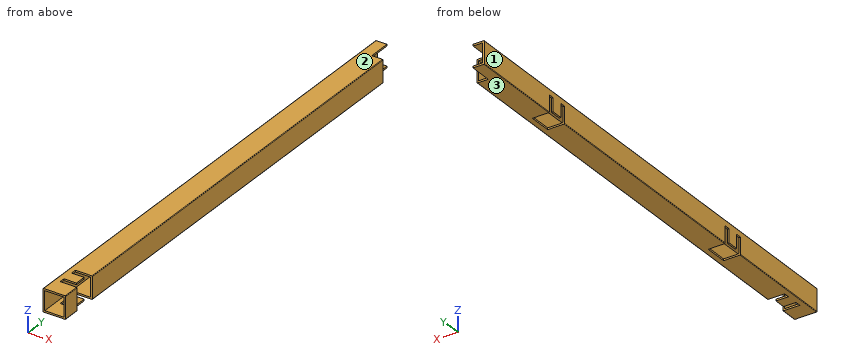
```python
from build123d import *

# Parameters (mm, degrees)
SKETCH1_W                   = 17
SKETCH1_H                   = 17
BOSS_EXTRUDE1_DEPTH         = 1220
SKETCH2_W                   = 20
SKETCH2_H                   = 20
CUT_EXTRUDE1_DEPTH          = 10
CUT_EXTRUDE2_DEPTH          = 15
SKETCH4_W                   = 3
SKETCH4_H                   = 10
CUT_EXTRUDE3_DEPTH          = 10
SKETCH_PATTERN1_START       = -20
SKETCH_PATTERN1_DEPTH       = 15
SKETCH_PATTERN1_2_OUTLINE_W = 1.5
SKETCH_PATTERN1_2_OUTLINE_H = 10
SKETCH_PATTERN1_2_DEPTH     = 3
SKETCH6_W                   = 20
SKETCH6_H                   = 20
CUT_EXTRUDE4_DEPTH          = 4
CUT_EXTRUDE5_DEPTH          = 1221.327824808
CUT_EXTRUDE5_DEPTH_BACK     = 1221.327824808
SKETCH7_W                   = 11
SKETCH7_H                   = 5
SKETCH8_W                   = 20.081282068
SKETCH8_H                   = 792.599518512
CUT_EXTRUDE6_DEPTH          = 20


# Read off the part's stored shape, not the designer's step: Sketch-Pattern1
with BuildPart() as part:
    # Sketch1 → Boss-Extrude1 (new body)
    with BuildSketch(Plane(origin=(0, 0, 0), x_dir=(1, 0, 0), z_dir=(0, 1, 0))):
        with BuildLine():
            Line((0.5, 0), (19.5, 0))
            ThreePointArc((19.5, 0), (19.853553391, 0.146446609), (20, 0.5))
            Line((20, 0.5), (20, 19.5))
            ThreePointArc((20, 19.5), (19.853553391, 19.853553391), (19.5, 20))
            Line((19.5, 20), (0.5, 20))
            ThreePointArc((0.5, 20), (0.146446609, 19.853553391), (0, 19.5))
            Line((0, 19.5), (0, 0.5))
            ThreePointArc((0, 0.5), (0.146446609, 0.146446609), (0.5, 0))
        make_face()
        with Locations((10, 10)):
            Rectangle(SKETCH1_W, SKETCH1_H, mode=Mode.SUBTRACT)
    extrude(amount=BOSS_EXTRUDE1_DEPTH)

    # Sketch2 → Cut-Extrude1 (cut)
    with BuildSketch(Plane(origin=(20, 0, 0), x_dir=(0, 0, -1), z_dir=(1, 0, 0))):
        with Locations((10, 1210)):
            Rectangle(SKETCH2_W, SKETCH2_H)
        with Locations((10, 10)):
            Rectangle(SKETCH2_W, SKETCH2_H)
    extrude(amount=-CUT_EXTRUDE1_DEPTH, mode=Mode.SUBTRACT)

    # Sketch3 → Cut-Extrude2 (cut)
    with BuildSketch(Plane(origin=(0, 0, -20), x_dir=(-1, 0, 0), z_dir=(0, 0, -1))):
        Polygon((-15, 1115), (0, 1115), (0, 1120), (-9, 1120), (-9, 1130), (0, 1130), (0, 1135), (-15, 1135), align=None)
    extrude(amount=-CUT_EXTRUDE2_DEPTH, mode=Mode.SUBTRACT)

    # Sketch4 → Cut-Extrude3 (cut)
    with BuildSketch(Plane.ZY):
        with Locations((-18.5, 1125)):
            Rectangle(SKETCH4_W, SKETCH4_H)
    extrude(amount=-CUT_EXTRUDE3_DEPTH, mode=Mode.SUBTRACT)

    # Sketch-Pattern1 outline → Sketch-Pattern1 (cut)
    with BuildSketch(Plane.XY.offset(SKETCH_PATTERN1_START)):
        Polygon((15, 105), (15, 125), (0, 125), (0, 120), (1.5, 120), (1.5, 110), (0, 110), (0, 105), align=None)
        Polygon((1.5, 350), (1.5, 340), (0, 340), (0, 335), (15, 335), (15, 355), (0, 355), (0, 350), align=None)
        Polygon((1.5, 510), (1.5, 500), (0, 500), (0, 495), (15, 495), (15, 515), (0, 515), (0, 510), align=None)
        Polygon((1.5, 740), (1.5, 730), (0, 730), (0, 725), (15, 725), (15, 745), (0, 745), (0, 740), align=None)
        Polygon((1.5, 900), (1.5, 890), (0, 890), (0, 885), (15, 885), (15, 905), (0, 905), (0, 900), align=None)
    extrude(amount=SKETCH_PATTERN1_DEPTH, mode=Mode.SUBTRACT)

    # Sketch-Pattern1 2 outline → Sketch-Pattern1 2 (cut)
    with BuildSketch(Plane.XY.offset(SKETCH_PATTERN1_START)):
        with Locations((0.75, 115)):
            Rectangle(SKETCH_PATTERN1_2_OUTLINE_W, SKETCH_PATTERN1_2_OUTLINE_H)
        with Locations((0.75, 345)):
            Rectangle(SKETCH_PATTERN1_2_OUTLINE_W, SKETCH_PATTERN1_2_OUTLINE_H)
        with Locations((0.75, 505)):
            Rectangle(SKETCH_PATTERN1_2_OUTLINE_W, SKETCH_PATTERN1_2_OUTLINE_H)
        with Locations((0.75, 735)):
            Rectangle(SKETCH_PATTERN1_2_OUTLINE_W, SKETCH_PATTERN1_2_OUTLINE_H)
        with Locations((0.75, 895)):
            Rectangle(SKETCH_PATTERN1_2_OUTLINE_W, SKETCH_PATTERN1_2_OUTLINE_H)
    extrude(amount=SKETCH_PATTERN1_2_DEPTH, mode=Mode.SUBTRACT)

    # Sketch6 → Cut-Extrude4 (cut)
    with BuildSketch(Plane(origin=(20, 0, 0), x_dir=(0, 0, -1), z_dir=(1, 0, 0))):
        with Locations((10, 810)):
            Rectangle(SKETCH6_W, SKETCH6_H)
    extrude(amount=-CUT_EXTRUDE4_DEPTH, mode=Mode.SUBTRACT)

    # Sketch7 → Cut-Extrude5 (cut, two sides: drawn at the far end of the back side and taken through both)
    with BuildSketch(Plane(origin=(0, 0, -20), x_dir=(-1, 0, 0), z_dir=(0, 0, -1)).offset(-CUT_EXTRUDE5_DEPTH_BACK)):
        with Locations((-10.5, 817.5)):
            Rectangle(SKETCH7_W, SKETCH7_H)
        with Locations((-10.5, 802.5)):
            Rectangle(SKETCH7_W, SKETCH7_H)
    extrude(amount=CUT_EXTRUDE5_DEPTH + CUT_EXTRUDE5_DEPTH_BACK, mode=Mode.SUBTRACT)

    # Sketch8 → Cut-Extrude6 (cut)
    with BuildSketch(Plane(origin=(0, 0, -20), x_dir=(-1, 0, 0), z_dir=(0, 0, -1))):
        with Locations((-10.040641034, 388.700240744)):
            Rectangle(SKETCH8_W, SKETCH8_H)
    extrude(amount=-CUT_EXTRUDE6_DEPTH, mode=Mode.SUBTRACT)


solid = part.part
```
For this review, take the finished solid that the model builds, in its own axes (mm). Face numbers are marked on the shaded views. Round coordinates to 2 decimals unless told otherwise and drop trailing zeros. Write each loop counter-clockwise with the first axis right and the second up, starting at its lowest first coordinate (ties: lowest second). Pieces come first, ordered by that corner, then holes. Notation, with made-up numbers: (-15, 74) -> (9, 74) arc R34 cw to (9, 105) -> close; hole circle Ø9 at (27, 83). An arc over 180 degrees is marked (long way). Use one line per item in the form item = value.
Q1. The part is to be moulded in two halves that separate along Z. For the marked faces 1, 2 and 3, say which applies: released by +Z, released by -Z, zero draft, split by the parting line, or undercut.
Resolved:
face_1 = zero draft
face_2 = released by +Z
face_3 = released by -Z
Q2. Consider section B-B (y = 967). State the section outline as (x, z) points.
Resolved:
outline = (0, -19.5) arc R0.5 ccw to (0.5, -20) -> (19.5, -20) arc R0.5 ccw to (20, -19.5) -> (20, -0.5) arc R0.5 ccw to (19.5, 0) -> (0.5, 0) arc R0.5 ccw to (0, -0.5) -> close; hole (1.5, -18.5) -> (18.5, -18.5) -> (18.5, -1.5) -> (1.5, -1.5) -> close
Q3. Clearance check with flat-ended pins moving along their axes: pin 1 Ø1.6 at (x, y) = (0.5, 887.5) entering from -Z; pin 2 Ø7.5 at (x, z) = (15, -6) entering from +Y; pin 3 Ø1 at (x, y) = (7.5, 895) entering from -Z; pin 4 Ø10 at (y, z) = (1067.5, -3) entering from -X. State where each tip first meets the part, or that it passes through.
Resolved:
pin_1 = -5
pin_2 = 1200
pin_3 = -1.5
pin_4 = 0
Q4. Consider section A-A (z = -13). State the section outline as (x, y) points, then the cut area to 4 significant figures.
Resolved:
outline = (0, 785) -> (1.5, 785) -> (1.5, 885) -> (0, 885) -> close; (0, 890) -> (1.5, 890) -> (1.5, 900) -> (0, 900) -> close; (0, 905) -> (1.5, 905) -> (1.5, 1115) -> (0, 1115) -> close; (0, 1120) -> (1.5, 1120) -> (1.5, 1130) -> (0, 1130) -> close; (0, 1135) -> (1.5, 1135) -> (1.5, 1220) -> (0, 1220) -> close; (18.5, 785) -> (20, 785) -> (20, 800) -> (18.5, 800) -> close; (18.5, 820) -> (20, 820) -> (20, 1200) -> (18.5, 1200) -> close
area = 1,215 mm²
Q5. To check wall thickness, follow probe 1 along Y at (x, z) = (9.25, -18.75); probe 2 along X at (y, z) = (1001.5, -13.75); probe 3 along Z at (x, y) = (12.25, 876.5). State the ranges of each line that lie inside material, in increasing order. Write a range as from..to.
Resolved:
probe_1 = 785..800, 805..815, 820..885, 905..1115, 1135..1220
probe_2 = 0..1.5, 18.5..20
probe_3 = -20..-18.5, -1.5..0
